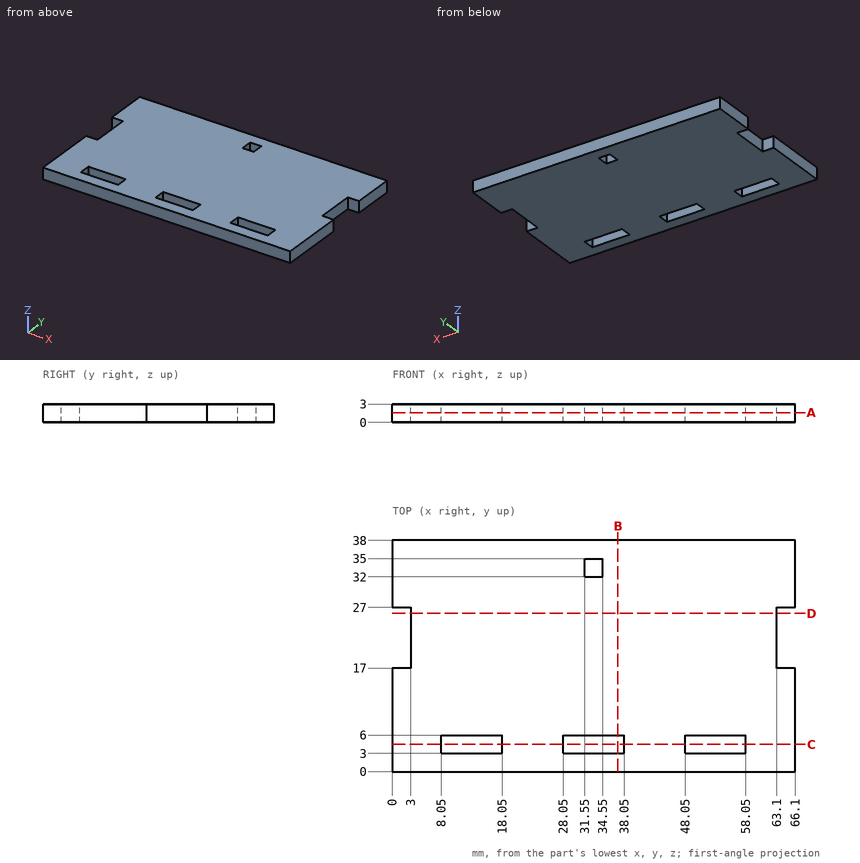
Study the drawing (mm; zero at the part's minimum x, y, z) and answer. Give positions to 0.01 mm unless a question says otherwise; leave off trailing zeros. Write each loop counter-clockwise with the first axis right and the second up, starting at its lowest first coordinate (ties: lowest second). Pieces come first, ordered by that corner, then holes. Notation, with made-up numbers: (78, -25) -> (82, -25) arc R26 ccw to (82, 10) -> close; hole circle Ø9 at (0.5, 71.25). An arc over 180 degrees is marked (long way). Write item = value, one per line. Start each with the question number.
1) The part is cut by section C-C, the plane y = 4.5. Determine the outline of the cut face in (x, z), and give its area (3 significant figures).
2) The part is cut by section B-B, the plane x = 37. Determine the outline of the cut face in (y, z).
3) The part is cut by section D-D, the plane y = 26. Determine the outline of the cut face in (x, z).
4) The part is cut by section A-A, the plane z = 1.6. Determine the outline of the cut face in (x, y), and give its area (3 significant figures).
5) Each of these flat-tipped pins is pushed along its axis until it touches: pin 1 (1.5 mm diameter, centred on y = 21, z = 1, fed in from -X); pin 2 (1.5 mm diameter, centred on y = 23.5, z = 1.5, fed in from +X). Where does it stop, or does it pass through?
6) Straight lines are drawn through the part: line 1 along X through (y, z) = (32.5, 1); line 2 along Y through (x, z) = (63.5, 0.3); line 3 along Y through (x, z) = (9, 0.35). For each, find the intervals that lie inside material, in ascending order.
Solutions:
q1.outline = (0, 0) -> (8.05, 0) -> (8.05, 3) -> (0, 3) -> close; (18.05, 0) -> (28.05, 0) -> (28.05, 3) -> (18.05, 3) -> close; (38.05, 0) -> (48.05, 0) -> (48.05, 3) -> (38.05, 3) -> close; (58.05, 0) -> (66.1, 0) -> (66.1, 3) -> (58.05, 3) -> close
q1.area = 108 mm²
q2.outline = (0, 0) -> (3, 0) -> (3, 3) -> (0, 3) -> close; (6, 0) -> (38, 0) -> (38, 3) -> (6, 3) -> close
q3.outline = (3, 0) -> (63.1, 0) -> (63.1, 3) -> (3, 3) -> close
q4.outline = (0, 0) -> (66.1, 0) -> (66.1, 17) -> (63.1, 17) -> (63.1, 27) -> (66.1, 27) -> (66.1, 38) -> (0, 38) -> (0, 27) -> (3, 27) -> (3, 17) -> (0, 17) -> close; hole (8.05, 3) -> (18.05, 3) -> (18.05, 6) -> (8.05, 6) -> close; hole (28.05, 3) -> (38.05, 3) -> (38.05, 6) -> (28.05, 6) -> close; hole (31.55, 32) -> (34.55, 32) -> (34.55, 35) -> (31.55, 35) -> close; hole (48.05, 3) -> (58.05, 3) -> (58.05, 6) -> (48.05, 6) -> close
q4.area = 2,350 mm²
q5.pin_1 = 3
q5.pin_2 = 63.1
q6.line_1 = 0 to 31.55, 34.55 to 66.1
q6.line_2 = 0 to 17, 27 to 38
q6.line_3 = 0 to 3, 6 to 38
